Input: part model. Units: mm. Frame: model coordinates. A direction names the side the tool comes from. Give positions to 0.01 mm unless a question says otherwise; leave off trailing zeros. Loops run counter-clockwise (first coordinate to the right, second up) from the corner with the lowest first, then second, coordinate; pieces in that order, holes last. Notation, with made-up numbers: (73, 33.5) - (129, 33.5) arc R29 cw to (129, 71.5) - close; hole circle Ø8 at (39.5, 74.5). An arc over 180 degrees is marked (long way). One line per question, with ' | ' between items. Start each with the question number.
from build123d import *

# Parameters (mm, degrees)
EXTRUDE_1_DEPTH     = 72.39
SKETCH_2_W          = 63.894569667
SKETCH_2_H          = 50.584743582
EXTRUDE_2_DEPTH     = 35.72348927
SKETCH_3_W          = 47.81706323
SKETCH_3_H          = 19.199275388
EXTRUDE_4_DEPTH     = 78.486
CUT_EXTRUDE_4_DEPTH = 22.098
SKETCH_7_W          = 85.131498904
SKETCH_7_H          = 43.590498022
CUT_EXTRUDE_5_DEPTH = 22.098
EXTRUDE_5_DEPTH     = 20.066


with BuildPart() as part:
    # 草图1 → 凸台-拉伸1 (new body)
    with BuildSketch(Plane.XY):
        Polygon((30.681441224, -0.764247788), (59.9139191, -0.764247788), (59.9139191, -29.041415929), (-40.202541077, -29.041415929), (-40.202541077, -0.764247788), (-40.202541077, 43.371061947), (30.681441224, 43.371061947), align=None)
    extrude(amount=EXTRUDE_1_DEPTH)

    # 草图2 → 凸台-拉伸2 (add)
    with BuildSketch(Plane(origin=(0, 43.371061947, 0), x_dir=(1, 0, 0), z_dir=(0, 1, 0))):
        with Locations((-1.26584361, 16.441925792)):
            Rectangle(SKETCH_2_W, SKETCH_2_H)
    extrude(amount=EXTRUDE_2_DEPTH)

    # 草图3 → 凸台-拉伸4 (add)
    with BuildSketch(Plane(origin=(0, 43.371061947, 0), x_dir=(1, 0, 0), z_dir=(0, 1, 0))):
        with Locations((5.873027985, -55.236552657)):
            Rectangle(SKETCH_3_W, SKETCH_3_H)
    extrude(amount=EXTRUDE_4_DEPTH)

    # 草图6 → 切除-拉伸4 (cut)
    with BuildSketch(Plane.XY.offset(64.836190351)):
        with BuildLine():
            Line((-18.03550363, 121.857061947), (-18.03550363, 96.233075723))
            ThreePointArc((-18.03550363, 96.233075723), (5.04667963, 120.12732257), (29.724437597, 97.884784986))
            Line((29.724437597, 97.884784986), (29.774943726, 121.857061947))
            Line((29.774943726, 121.857061947), (-18.03550363, 121.857061947))
        make_face()
    extrude(amount=-CUT_EXTRUDE_4_DEPTH, mode=Mode.SUBTRACT)

    # 草图7 → 切除-拉伸5 (cut)
    with BuildSketch(Plane(origin=(0, 0, -41.734297583), x_dir=(-1, 0, 0), z_dir=(0, 0, -1))):
        with Locations((8.884308228, 58.531001223)):
            Rectangle(SKETCH_7_W, SKETCH_7_H)
    extrude(amount=-CUT_EXTRUDE_5_DEPTH, mode=Mode.SUBTRACT)

    # 草图8 → 凸台-拉伸5 (add)
    with BuildSketch(Plane(origin=(0, 0, -19.636297583), x_dir=(-1, 0, 0), z_dir=(0, 0, -1))):
        with BuildLine():
            ThreePointArc((1.878708632, 90.752463726), (-10.775595888, 102.192073522), (-22.633627477, 89.928991445))
            Line((-22.633627477, 89.928991445), (-22.633627477, 79.094551217))
            Line((-22.633627477, 79.094551217), (-12.26491781, 79.094551217))
            ThreePointArc((-12.26491781, 79.094551217), (-17.43772835, 98.352594999), (0.636372523, 89.928991445))
            ThreePointArc((0.636372523, 89.928991445), (-1.940023923, 82.854890572), (-8.462337143, 79.094551217))
            Line((-8.462337143, 79.094551217), (1.899704254, 79.094551217))
            Line((1.899704254, 79.094551217), (1.881595314, 89.149620673))
            Line((1.881595314, 89.149620673), (1.878708632, 90.752463726))
        make_face()
        with BuildLine():
            Line((-12.26491781, 79.094551217), (-22.633627477, 79.094551217))
            Line((-22.633627477, 79.094551217), (-22.633627477, 75.391965029))
            Line((-22.633627477, 75.391965029), (1.906372523, 75.391965029))
            Line((1.906372523, 75.391965029), (1.899704254, 79.094551217))
            Line((1.899704254, 79.094551217), (-8.462337143, 79.094551217))
            ThreePointArc((-8.462337143, 79.094551217), (-10.363627477, 78.928991445), (-12.26491781, 79.094551217))
        make_face()
    extrude(amount=-EXTRUDE_5_DEPTH)


solid = part.part
Q1. Access query for faces 4 (the face through (-18.036, 69, 55)), 5 (the face through (-1, 8, 0)), 6 (the face through (10.5, 102.2, -9.7)), 7 (the face through (22.634, 85, -10)), 8 (the face through (45, -0.764, 36)). Directions: +Z, -Z, +X, -X, +Y, -Y. A direction counts if a zero-diameter tool reaches every point of the face in a straight line with its end or side. Return the directions, or none.
Q2. Section A-A, the plane y = 68. Output: boundary loops of the cut face in (x, z).
Q3. Section B-B, the plane x = 3. Output: boundary loops of the cut face in (y, z).
Q4. First-contact query: pin 1 (21 mm diameter, centred on y = 76.5, z = 51, fed in from +X); pin 2 (10 mm diameter, centred on x = -2, z = -6, fed in from -Y); pin 3 (10 mm diameter, centred on x = -12.5, y = 93, fed in from +Z). Flat tips, straight axial feed; report the tip coordinate or a pass-through.
Q5. Draft query along X for faces 1 (the face through (4.533, 120.104, 55.371)), 2 (the face through (6, 82, 64.836)), 3 (the face through (29.782, 82, 55)). Return one class per face: +X half, -X half, draft (parallel to the pull), parting line (faces both ways), or undercut.
Q6. Section C-C, the plane z = -5.5. Output: boundary loops of the cut face in (x, y), plus the area to 4 significant figures.
Q7. Section D-D, the plane x = -27.5. Output: boundary loops of the cut face in (y, z).
Q8. Line query: L1, parallel to Z at x = -11.5, y = 72; L2, parallel to Z at x = -32, y = -19; L3, parallel to Y at x = -0.5, z = 35. Output: solid intervals per line, ascending. Write a range as from..to.
Solved:
1) face 4: +Z, -X, +Y | face 5: -Z, +X, -X, -Y | face 6: -Z, +Y | face 7: -Z, +X, +Y | face 8: +Z, -Z, +X, +Y
2) outline: (-33.21, -19.64) - (30.68, -19.64) - (30.68, 8.85) - (-33.21, 8.85) - close; (-18.04, 45.64) - (29.78, 45.64) - (29.78, 64.84) - (-18.04, 64.84) - close
3) outline: (-29.04, 0) - (43.37, 0) - (43.37, -19.64) - (81.76, -19.64) - (81.76, 0.43) - (79.09, 0.43) - (79.09, 8.85) - (43.37, 8.85) - (43.37, 45.64) - (119.97, 45.64) - (119.97, 64.84) - (43.37, 64.84) - (43.37, 72.39) - (-29.04, 72.39) - close; (98.1, -19.64) - (99.74, -19.64) - (99.74, 0.43) - (98.1, 0.43) - close
4) pin 1: stops at x = 29.78 | pin 2: stops at y = 43.37 | pin 3: stops at z = 64.84
5) face 1: undercut | face 2: draft | face 3: +X half
6) outline: (-33.21, 43.37) - (30.68, 43.37) - (30.68, 79.09) - (22.63, 79.09) - (22.63, 89.93) arc R12.27 ccw to (-1.88, 90.75) - (-1.9, 79.09) - (-33.21, 79.09) - close; hole (8.46, 79.09) - (12.26, 79.09) arc R11 ccw (long way) to start | area: 2,405 mm²
7) outline: (-29.04, 0) - (43.37, 0) - (43.37, -19.64) - (79.09, -19.64) - (79.09, 8.85) - (43.37, 8.85) - (43.37, 72.39) - (-29.04, 72.39) - close
8) L1: z = -19.64..8.85, 45.64..64.84 | L2: z = 0..72.39 | L3: y = -29.04..43.37
